from build123d import *

# Parameters (mm, degrees)
SKETCH1_W           = 38.1
SKETCH1_H           = 20.955
BOSS_EXTRUDE1_DEPTH = 56.515
FILLET1_R           = 3.175
SKETCH2_R           = 10.4775
BOSS_EXTRUDE2_DEPTH = 10.414


with BuildPart() as part:
    # Sketch1 → Boss-Extrude1 (new body)
    with BuildSketch(Plane(origin=(0, 0, 0), x_dir=(1, 0, 0), z_dir=(0, 1, 0))):
        Rectangle(SKETCH1_W, SKETCH1_H)
    extrude(amount=BOSS_EXTRUDE1_DEPTH)

    # Fillet1
    fillet1_edges = [part.edges().sort_by_distance(p)[0] for p in [
        (-19.05, 56.515, 0),
        (19.05, 56.515, 0),
        (-19.05, 0, 0),
        (19.05, 0, 0),
    ]]
    fillet(fillet1_edges, radius=FILLET1_R)

    # Sketch2 → Boss-Extrude2 (add)
    with BuildSketch(Plane(origin=(0, 56.515, 0), x_dir=(1, 0, 0), z_dir=(0, 1, 0))):
        Circle(SKETCH2_R)
    extrude(amount=BOSS_EXTRUDE2_DEPTH)


solid = part.part
Can you work these out from the model? Positions are in its coordinate system, mm. A direction names the side the tool comes from. Coordinates: 2 decimals unless noted, no trailing zeros. Loops run counter-clockwise (first coordinate to the right, second up) from the corner with the lowest first, then second, coordinate; pieces in that order, holes last. Notation, with made-up numbers: M 30,-0.5 L 70,-0.5 A12 cw 70,10.5 Z; hole C -33.5,1 d4. An arc over 180 degrees is marked long. Answer as CSV lines item,"result". Start each with the question number.
1. Suppose I cut it at D-D, the plane x = -14. List the corners of the cut face in (y, z) for me (1 decimal), plus the area to 3 significant figures.
2. For faces 1 (the face through (-1.36, 61.65, -10.39)), 2 (the face through (0, 28, -10.478)), 3 (the face through (11, 56.515, 0)), 4 (the face through (-12, 56.515, 0)), which set-ups out of +Z, -Z, +X, -X, +Y, -Y let a thin tool reach every point of the face, with its end or its side?
3. Suppose I cut it at C-C, the plane z = 7.5. List the corners of the cut face in (x, y) for me (3 decimals).
4. Suppose I cut it at B-B, the plane x = 4.5. List the corners of the cut face in (y, z) for me (1 decimal), plus the area to 3 significant figures.
5. If I drill on probe 1 along Y at (x, z) = (15, -3.25) (3 decimals); probe 2 along X at (y, z) = (58.5, -5.75); probe 3 along X at (y, z) = (59.5, 8), over which ranges is the centre line in solid material (lowest first)? Write a range as [from, to].
Output:
1,outline,"M 0,-10.5 L 56.5,-10.5 L 56.5,10.5 L 0,10.5 Z"
1,area,"1,180 mm^2"
2,face 1,"+Y"
2,face 2,"-Z, +X, -X, +Y, -Y"
2,face 3,"+X, +Y"
2,face 4,"-X, +Y"
3,outline,"M -19.05,3.175 A3.175 ccw -15.875,0 L 15.875,0 A3.175 ccw 19.05,3.175 L 19.05,53.34 A3.175 ccw 15.875,56.515 L 7.316,56.515 L 7.316,66.929 L -7.316,66.929 L -7.316,56.515 L -15.875,56.515 A3.175 ccw -19.05,53.34 Z"
4,outline,"M 0,-10.5 L 56.5,-10.5 L 56.5,-9.5 L 66.9,-9.5 L 66.9,9.5 L 56.5,9.5 L 56.5,10.5 L 0,10.5 Z"
4,area,"1,380 mm^2"
5,probe 1,"y = [0, 56.515]"
5,probe 2,"x = [-8.76, 8.76]"
5,probe 3,"x = [-6.77, 6.77]"
